from build123d import *

# Parameters (mm, degrees)
CROQUIS1_R              = 13.75
SALIENTE_EXTRUIR1_DEPTH = 12.5
CROQUIS2_R              = 15
SALIENTE_EXTRUIR2_DEPTH = 19.7
CROQUIS3_R              = 13.75
SALIENTE_EXTRUIR3_DEPTH = 5
CROQUIS4_R              = 5
SALIENTE_EXTRUIR4_DEPTH = 2.5
CROQUIS5_R              = 1.15
SALIENTE_EXTRUIR5_DEPTH = 2
CROQUIS6_R              = 4.4
SALIENTE_EXTRUIR6_DEPTH = 1.2
CROQUIS7_R              = 3.35
SALIENTE_EXTRUIR7_DEPTH = 5


with BuildPart() as part:
    # Croquis1 → Saliente-Extruir1 (new body)
    with BuildSketch(Plane(origin=(0, 0, 0), x_dir=(1, 0, 0), z_dir=(0, 1, 0))):
        Circle(CROQUIS1_R)
    extrude(amount=SALIENTE_EXTRUIR1_DEPTH)

    # Croquis2 → Saliente-Extruir2 (add)
    with BuildSketch(Plane(origin=(0, 12.5, 0), x_dir=(1, 0, 0), z_dir=(0, 1, 0))):
        Circle(CROQUIS2_R)
    extrude(amount=SALIENTE_EXTRUIR2_DEPTH)

    # Croquis3 → Saliente-Extruir3 (add)
    with BuildSketch(Plane(origin=(0, 32.2, 0), x_dir=(1, 0, 0), z_dir=(0, 1, 0))):
        Circle(CROQUIS3_R)
    extrude(amount=SALIENTE_EXTRUIR3_DEPTH)

    # Croquis4 → Saliente-Extruir4 (add)
    with BuildSketch(Plane(origin=(0, 37.2, 0), x_dir=(1, 0, 0), z_dir=(0, 1, 0))):
        Circle(CROQUIS4_R)
    extrude(amount=SALIENTE_EXTRUIR4_DEPTH)

    # Croquis5 → Saliente-Extruir5 (add)
    with BuildSketch(Plane(origin=(0, 39.7, 0), x_dir=(1, 0, 0), z_dir=(0, 1, 0))):
        Circle(CROQUIS5_R)
    extrude(amount=SALIENTE_EXTRUIR5_DEPTH)

    # Croquis6 → Saliente-Extruir6 (add)
    with BuildSketch(Plane(origin=(0, 41.7, 0), x_dir=(1, 0, 0), z_dir=(0, 1, 0))):
        Circle(CROQUIS6_R)
    extrude(amount=SALIENTE_EXTRUIR6_DEPTH)

    # Croquis7 → Saliente-Extruir7 (add)
    with BuildSketch(Plane(origin=(0, 42.9, 0), x_dir=(1, 0, 0), z_dir=(0, 1, 0))):
        Circle(CROQUIS7_R)
    extrude(amount=SALIENTE_EXTRUIR7_DEPTH)


solid = part.part
CAD build for the part. Positions are in the model's coordinates, mm. A direction names the side the tool comes from. Round coordinates to 2 decimals unless told otherwise and drop trailing zeros. Write each loop counter-clockwise with the first axis right and the second up, starting at its lowest first coordinate (ties: lowest second). Pieces come first, ordered by that corner, then holes.
(1) Slice it at A-A, the plane z = 0. Write the cut outline in (x, y), and give its area (3 significant figures).
(2) Slice it at C-C, the plane y = 9. Write the cut outline in (x, z), and give its area (3 significant figures).
(3) Drop flat-ended pins along their axis: P1, Ø5, axis at x = 8, z = 10.5, coming from the +Y side; P2, Ø2, axis at x = -9, y = 23.5, coming from the -Z side; P3, Ø6, axis at x = -7.5, z = -1.5, coming from the +Y side. Give the stop position or say it passes through.
(4) Slice it at D-D, the plane z = -12.5. Write the cut outline in (x, y), and give its area (3 significant figures).
(5) 3-axis set-ups, long thin cutter, end or side, ignore diameter. For faces 1 (the face through (-3.347, 45.365, -0.147)), 2 (the face through (1, 41.7, 1)), 3 (the face through (4.4, 12.5, 13.3)): which of +Z, -Z, +X, -X, +Y, -Y reach the whole face in a straight line?
(6) Probe line 1 along Y through (x, z) = (0.5, 4); line 2 along Y through (x, z) = (-3, 11.25); line 3 along Z through (x, y) = (1.25, 42.5). List the from-to ranges inside material, lowest first.
(7) Slice it at B-B, the plane x = 0. Write the cut outline in (y, z), and give its area (3 significant figures).
(8) Mould opens along Y. For faces 4 (the face through (4.197, 42.292, -1.322)), 5 (the face through (4.4, 32.2, 13.3)), 6 (the face through (1, 39.7, 1)) say: pulls with the +Y half, pulls with the -Y half, needs draft (parallel to the pull), parting line crosses it, or undercut.
From the geometry:
1. outline: (-15, 12.5) - (-13.75, 12.5) - (-13.75, 0) - (13.75, 0) - (13.75, 12.5) - (15, 12.5) - (15, 32.2) - (13.75, 32.2) - (13.75, 37.2) - (5, 37.2) - (5, 39.7) - (1.15, 39.7) - (1.15, 41.7) - (4.4, 41.7) - (4.4, 42.9) - (3.35, 42.9) - (3.35, 47.9) - (-3.35, 47.9) - (-3.35, 42.9) - (-4.4, 42.9) - (-4.4, 41.7) - (-1.15, 41.7) - (-1.15, 39.7) - (-5, 39.7) - (-5, 37.2) - (-13.75, 37.2) - (-13.75, 32.2) - (-15, 32.2) - close
1. area: 1,150 mm2
2. outline: circle Ø27.5 at (0, 0)
2. area: 594 mm2
3. P1: stops at y = 37.2
3. P2: stops at z = -12.69
3. P3: stops at y = 39.7
4. outline: (-8.29, 12.5) - (-5.73, 12.5) - (-5.73, 0) - (5.73, 0) - (5.73, 12.5) - (8.29, 12.5) - (8.29, 32.2) - (5.73, 32.2) - (5.73, 37.2) - (-5.73, 37.2) - (-5.73, 32.2) - (-8.29, 32.2) - close
4. area: 527 mm2
5. face 1: +Y
5. face 2: none
5. face 3: -Y
6. line 1: y = 0 to 39.7, 41.7 to 42.9
6. line 2: y = 0 to 37.2
6. line 3: z = -4.22 to 4.22
7. outline: (0, -13.75) - (12.5, -13.75) - (12.5, -15) - (32.2, -15) - (32.2, -13.75) - (37.2, -13.75) - (37.2, -5) - (39.7, -5) - (39.7, -1.15) - (41.7, -1.15) - (41.7, -4.4) - (42.9, -4.4) - (42.9, -3.35) - (47.9, -3.35) - (47.9, 3.35) - (42.9, 3.35) - (42.9, 4.4) - (41.7, 4.4) - (41.7, 1.15) - (39.7, 1.15) - (39.7, 5) - (37.2, 5) - (37.2, 13.75) - (32.2, 13.75) - (32.2, 15) - (12.5, 15) - (12.5, 13.75) - (0, 13.75) - close
7. area: 1,150 mm2
8. face 4: needs draft
8. face 5: pulls with the +Y half
8. face 6: undercut
